from build123d import *

# Parameters (mm, degrees)
MODEL_R                  = 3.05
MODEL_R_2                = 2.55
BODY_DEPTH               = 6
SKETCH1_R                = 1.75
FORSENSOR_DEPTH          = 10
F_5_1_5_1_FOOTINGMOUNT_D = 5.1


with BuildPart() as part:
    # Model → Body (new body)
    with BuildSketch(Plane.XY):
        with BuildLine():
            Line((59.121320344, 14.121320344), (45.878679656, 0.878679656))
            ThreePointArc((45.878679656, 0.878679656), (44.90540961, 0.228361402), (43.757359313, 0))
            Line((43.757359313, 0), (3, 0))
            ThreePointArc((3, 0), (0.878679656, 0.878679656), (0, 3))
            Line((0, 3), (0, 82))
            ThreePointArc((0, 82), (0.878679656, 84.121320344), (3, 85))
            Line((3, 85), (19.471019058, 85))
            ThreePointArc((19.471019058, 85), (19.991963591, 84.954423259), (20.497079488, 84.819077862))
            Line((20.497079488, 84.819077862), (58.02606043, 71.159645877))
            ThreePointArc((58.02606043, 71.159645877), (59.457456133, 70.061297324), (60, 68.340568015))
            Line((60, 68.340568015), (60, 16.242640687))
            ThreePointArc((60, 16.242640687), (59.771638598, 15.09459039), (59.121320344, 14.121320344))
        make_face()
        with Locations((10, 75)):
            Circle(MODEL_R, mode=Mode.SUBTRACT)
        with Locations((10, 55)):
            Circle(MODEL_R, mode=Mode.SUBTRACT)
        with Locations((30, 55)):
            Circle(MODEL_R_2, mode=Mode.SUBTRACT)
        with Locations((50, 55)):
            Circle(MODEL_R_2, mode=Mode.SUBTRACT)
        with BuildLine():
            Line((12.5, 63.25), (7.5, 63.25))
            ThreePointArc((7.5, 63.25), (5.75, 65), (7.5, 66.75))
            Line((7.5, 66.75), (12.5, 66.75))
            ThreePointArc((12.5, 66.75), (14.25, 65), (12.5, 63.25))
        make_face(mode=Mode.SUBTRACT)
    extrude(amount=BODY_DEPTH)

    # Sketch1 → ForSensor (cut)
    with BuildSketch(Plane(origin=(0, 0, 0), x_dir=(-1, 0, 0), z_dir=(0, 0, -1))):
        with Locations((-10, 30)):
            Circle(SKETCH1_R)
        with Locations((-10, 37.5)):
            Circle(SKETCH1_R)
    extrude(amount=-FORSENSOR_DEPTH, mode=Mode.SUBTRACT)

    # Ø5.1 (5.1) FootingMount (through all)
    with Locations(Plane.XY.offset(6)):
        with Locations((25, 10), (25, 30)):
            Hole(F_5_1_5_1_FOOTINGMOUNT_D / 2)


solid = part.part
Read the model definition and answer for the solid it produces. Units are mm, in the model's axes. A direction names the side the tool comes from. Round coordinates to 2 decimals unless told otherwise and drop trailing zeros. Order: outer loops, then holes, each group sorted by start corner. A loop starts at its lowest first (then second) coordinate and runs counter-clockwise, first axis right, second up. Notation, with made-up numbers: (33.25, 10.5) - (60.25, 10.5) arc R11 ccw to (60.25, 15.5) - close; hole circle Ø8 at (27.25, 79). An arc over 180 degrees is marked (long way). Use one line per item in the form item = value. Start each with the question number.
(1) Find the intervals of material crossed by line 1 along Y through (x, z) = (25, 4.75); line 2 along Y through (x, z) = (10, 2.5); line 3 along Y through (x, z) = (26.5, 3.6), in increasing order. Write a range as from..to.
(2) The part is cut by section C-C (y = 37.5). Give the vertices of the cut face in (x, z), then the cut area to 3 significant figures.
(3) The part is cut by section D-D (x = 25). Give the vertices of the cut face in (y, z), then the cut area to 3 significant figures.
(4) The part is cut by section A-A (y = 55). Give the vertices of the cut face in (x, z), then the cut area to 3 significant figures.
(5) The part is cut by section B-B (z = 2.05). Count the separate pieces of the cut face and the enclosed holes in it, then the cut area to 3 significant figures.
(6) Determine the mould class of faces 1 (the face through (0.86, 84.1, 2.96)), 2 (the face through (59.78, 15.11, 2.96)), 3 (the face through (5.75, 64.96, 2.96)) for opening direction X: +X half, -X half, draft (parallel to the pull), parting line (faces both ways), or undercut.
(7) For faces 4 (the face through (14.25, 65.04, 2.96)), 5 (the face through (60, 43, 3)), determine the directions among +Z, -Z, +X, -X, +Y, -Y from which every point of the face is accessible in a straight line to the end or side of a thin tool.
(8) Flat-ended cylindrical pins translate along their axes: pin 1 Ø3 at (x, y) = (10, 37.5) entering from +Z; pin 2 Ø1.5 at (x, z) = (22.5, 2) entering from +Y. Find the tip coordinate at first contact, or state that the pin passes through.
Checked values:
q1.line_1 = 0..7.45, 12.55..27.45, 32.55..83.18
q1.line_2 = 0..28.25, 31.75..35.75, 39.25..51.95, 58.05..63.25, 66.75..71.95, 78.05..85
q1.line_3 = 0..7.94, 12.06..27.94, 32.06..82.63
q2.outline = (0, 0) - (8.25, 0) - (8.25, 6) - (0, 6) - close; (11.75, 0) - (60, 0) - (60, 6) - (11.75, 6) - close
q2.area = 339 mm^2
q3.outline = (0, 0) - (7.45, 0) - (7.45, 6) - (0, 6) - close; (12.55, 0) - (27.45, 0) - (27.45, 6) - (12.55, 6) - close; (32.55, 0) - (83.18, 0) - (83.18, 6) - (32.55, 6) - close
q3.area = 438 mm^2
q4.outline = (0, 0) - (6.95, 0) - (6.95, 6) - (0, 6) - close; (13.05, 0) - (27.45, 0) - (27.45, 6) - (13.05, 6) - close; (32.55, 0) - (47.45, 0) - (47.45, 6) - (32.55, 6) - close; (52.55, 0) - (60, 0) - (60, 6) - (52.55, 6) - close
q4.area = 262 mm^2
q5.separate_pieces = 1
q5.enclosed_holes = 9
q5.area = 4,500 mm^2
q6.face_1 = -X half
q6.face_2 = +X half
q6.face_3 = undercut
q7.face_4 = +Z, -Z
q7.face_5 = +Z, -Z, +X, +Y, -Y
q8.pin_1 = through
q8.pin_2 = 84.36
